Can you work these out from the drawing? Everything is in mm from the part's minimum corner. A direction names the side the tool comes from. Give positions to 0.01 mm unless a question says otherwise; leave off trailing zeros. Order: outer loops, then holes, each group sorted by start corner. A loop starts at its lowest first (then second) coordinate and runs counter-clockwise, first axis right, second up. Notation, with made-up numbers: M 41.5,36 L 90.5,36 A26 cw 90.5,62 Z; hole C -40,72.5 d5. An arc over 180 degrees is marked long. Use a Markdown table: item, result. Add a question column.
Item 1: If I drill on L1, parallel to Z at x = 47, y = 32; L2, parallel to Z at x = 23, y = 47.5; L3, parallel to X at y = 39, z = 26.5, over which ranges is the centre line in solid material (lowest first)? Write a range as from..to.
Item 2: Suppose I cut it at B-B on y = 4. Write out the boundary of the cut face in (x, z), plus the area to 3 significant figures.
Item 3: Suppose I cut it at C-C on z = 18. Write out the boundary of the cut face in (x, y).
Item 4: For the marked faces 1, 2 and 3, which set-ups out of +Z, -Z, +X, -X, +Y, -Y let a thin tool reach every point of the face, with its end or its side?
Item 5: I'm going to push flat-ended pins straight in: pin 1 Ø6 at (x, z) = (24, 31) entering from +Y; pin 2 Ø5 at (y, z) = (38.5, 23) entering from -X; pin 3 Ø8 at (x, y) = (15, 47) entering from +Z. Where does each tip first touch, or does it pass through?
Item 6: Suppose I cut it at A-A on x = 55.5. Write out the boundary of the cut face in (y, z), plus the area to 3 significant figures.
Item 7: Suppose I cut it at D-D on x = 19.5. Write out the boundary of the cut face in (y, z).
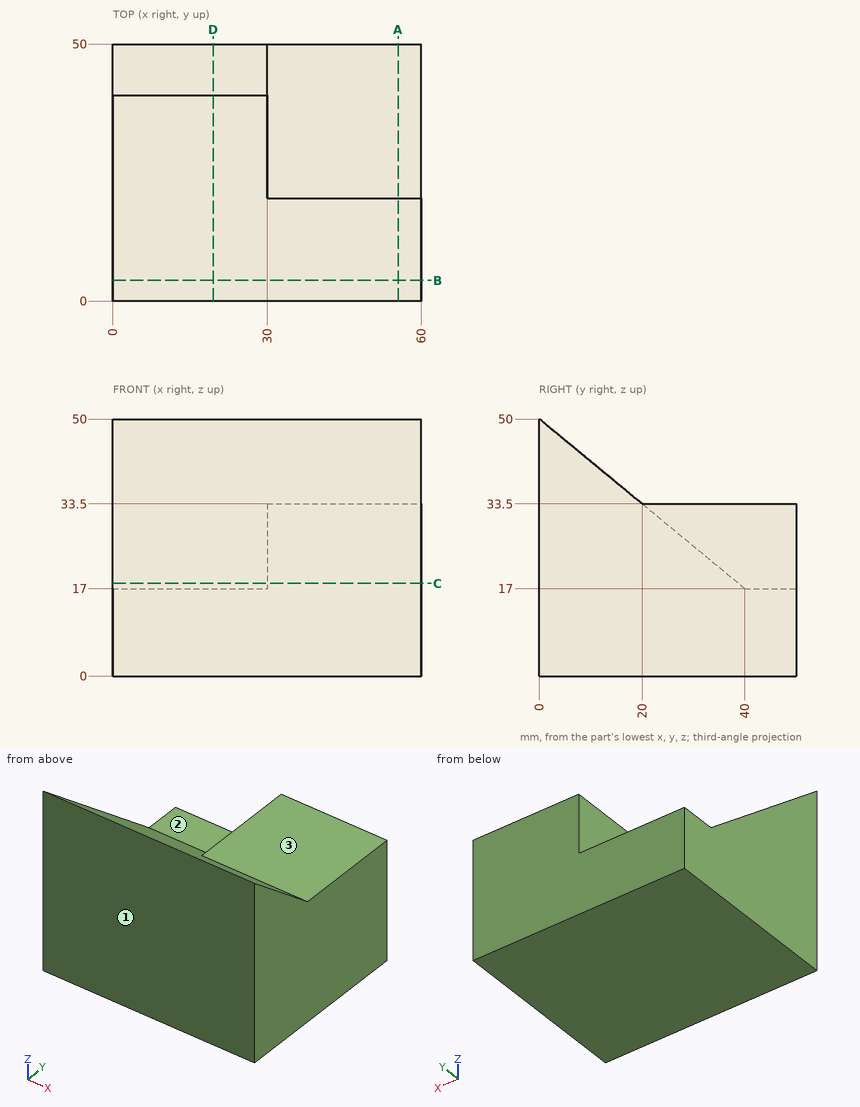
Findings below:
| question | item | result |
|---|---|---|
| 1 | L1 | z = 0..33.5 |
| 1 | L2 | z = 0..17 |
| 1 | L3 | x = 30..60 |
| 2 | outline | M 0,0 L 60,0 L 60,46.7 L 0,46.7 Z |
| 2 | area | 2,800 mm^2 |
| 3 | outline | M 0,0 L 60,0 L 60,50 L 30,50 L 30,38.79 L 0,38.79 Z |
| 4 | face 1 | +Z, -Z, +X, -X, -Y |
| 4 | face 2 | +Z, -X, +Y |
| 4 | face 3 | +Z, +X, -X, +Y |
| 5 | pin 1 | stops at y = 26.67 |
| 5 | pin 2 | stops at x = 30 |
| 5 | pin 3 | stops at z = 17 |
| 6 | outline | M 0,0 L 50,0 L 50,33.5 L 20,33.5 L 0,50 Z |
| 6 | area | 1,840 mm^2 |
| 7 | outline | M 0,0 L 50,0 L 50,17 L 40,17 L 0,50 Z |
